from build123d import *

# Parameters (mm, degrees)
SKETCH1_W           = 95.25
SKETCH1_H           = 247.65
BOSS_EXTRUDE1_DEPTH = 6.35
SKETCH2_R           = 38.1
CUT_EXTRUDE1_DEPTH  = 7.35
SKETCH3_W           = 6.35
SKETCH3_H           = 12.7
CUT_EXTRUDE2_DEPTH  = 7.35
LPATTERN1_COUNT     = 6
LPATTERN1_PITCH     = 25.4
SKETCH4_W           = 12.7
SKETCH4_H           = 6.35
CUT_EXTRUDE3_DEPTH  = 7.35
SKETCH5_W           = 12.7
SKETCH5_H           = 6.35
CUT_EXTRUDE4_DEPTH  = 7.35
SKETCH8_W           = 12.7
SKETCH8_H           = 6.881389346
CUT_EXTRUDE5_DEPTH  = 7.35
SKETCH9_R           = 1.75
CUT_EXTRUDE6_DEPTH  = 7.35
CIRPATTERN1_COUNT   = 4
FILLET1_R           = 12.7
SKETCH10_R          = 1.75
CUT_EXTRUDE7_DEPTH  = 7.35
CIRPATTERN2_COUNT   = 4


with BuildPart() as part:
    # Sketch1 → Boss-Extrude1 (new body)
    with BuildSketch(Plane(origin=(0, 0, 0), x_dir=(1, 0, 0), z_dir=(0, 1, 0))):
        with Locations((47.625, 123.825)):
            Rectangle(SKETCH1_W, SKETCH1_H)
    extrude(amount=BOSS_EXTRUDE1_DEPTH)

    # Sketch2 → Cut-Extrude1 (cut, through all)
    with BuildSketch(Plane(origin=(0, 6.35, 0), x_dir=(1, 0, 0), z_dir=(0, 1, 0))):
        with Locations((47.625, 200.025)):
            Circle(SKETCH2_R)
        with Locations((47.625, 47.625)):
            Circle(SKETCH2_R)
    extrude(amount=-CUT_EXTRUDE1_DEPTH, mode=Mode.SUBTRACT)

    # Sketch3 → Cut-Extrude2 (cut, through all)
    with BuildSketch(Plane(origin=(0, 6.35, 0), x_dir=(1, 0, 0), z_dir=(0, 1, 0))):
        with Locations((3.175, 6.35)):
            Rectangle(SKETCH3_W, SKETCH3_H)
        with Locations((92.075, 6.35)):
            Rectangle(SKETCH3_W, SKETCH3_H)
    cut_extrude2 = extrude(amount=-CUT_EXTRUDE2_DEPTH, mode=Mode.SUBTRACT)

    # LPattern1: Cut-Extrude2 ×6
    with Locations(*[(0, 0, -i * LPATTERN1_PITCH) for i in range(1, LPATTERN1_COUNT)]):
        add(cut_extrude2, mode=Mode.SUBTRACT)

    # Sketch4 → Cut-Extrude3 (cut, through all)
    with BuildSketch(Plane(origin=(0, 6.35, 0), x_dir=(1, 0, 0), z_dir=(0, 1, 0))):
        with Locations((47.625, 3.175)):
            Rectangle(SKETCH4_W, SKETCH4_H)
        with Locations((22.225, 3.175)):
            Rectangle(SKETCH4_W, SKETCH4_H)
        with Locations((73.025, 3.175)):
            Rectangle(SKETCH4_W, SKETCH4_H)
    extrude(amount=-CUT_EXTRUDE3_DEPTH, mode=Mode.SUBTRACT)

    # Sketch5 → Cut-Extrude4 (cut, through all)
    with BuildSketch(Plane(origin=(0, 6.35, 0), x_dir=(1, 0, 0), z_dir=(0, 1, 0))):
        with Locations((22.225, 92.075)):
            Rectangle(SKETCH5_W, SKETCH5_H)
        with Locations((47.625, 92.075)):
            Rectangle(SKETCH5_W, SKETCH5_H)
        with Locations((73.025, 92.075)):
            Rectangle(SKETCH5_W, SKETCH5_H)
    extrude(amount=-CUT_EXTRUDE4_DEPTH, mode=Mode.SUBTRACT)

    # Sketch8 → Cut-Extrude5 (cut, through all)
    with BuildSketch(Plane(origin=(0, 6.35, 0), x_dir=(1, 0, 0), z_dir=(0, 1, 0))):
        with Locations((22.225, 116.170967205)):
            Rectangle(SKETCH8_W, SKETCH8_H)
        with Locations((47.625, 116.170967205)):
            Rectangle(SKETCH8_W, SKETCH8_H)
        with Locations((73.025, 116.170967205)):
            Rectangle(SKETCH8_W, SKETCH8_H)
    extrude(amount=-CUT_EXTRUDE5_DEPTH, mode=Mode.SUBTRACT)

    # Sketch9 → Cut-Extrude6 (cut, through all)
    with BuildSketch(Plane(origin=(0, 6.35, 0), x_dir=(1, 0, 0), z_dir=(0, 1, 0))):
        with Locations((12.7, 82.55)):
            Circle(SKETCH9_R)
    cut_extrude6 = extrude(amount=-CUT_EXTRUDE6_DEPTH, mode=Mode.SUBTRACT)

    # CirPattern1: Cut-Extrude6 ×4 about axis
    cirpattern1_axis = Axis((47.625, 0, -47.625), (0, 1, 0))
    for i in range(1, CIRPATTERN1_COUNT):
        add(cut_extrude6.rotate(cirpattern1_axis, i * 360 / CIRPATTERN1_COUNT), mode=Mode.SUBTRACT)

    # Fillet1
    fillet1_edges = [part.edges().sort_by_distance(p)[0] for p in [
        (0, 3.175, -247.65),
        (95.25, 3.175, -247.65),
    ]]
    fillet(fillet1_edges, radius=FILLET1_R)

    # Sketch10 → Cut-Extrude7 (cut, through all)
    with BuildSketch(Plane(origin=(0, 6.35, 0), x_dir=(1, 0, 0), z_dir=(0, 1, 0))):
        with Locations((12.7, 234.95)):
            Circle(SKETCH10_R)
    cut_extrude7 = extrude(amount=-CUT_EXTRUDE7_DEPTH, mode=Mode.SUBTRACT)

    # CirPattern2: Cut-Extrude7 ×4 about axis
    cirpattern2_axis = Axis((47.625, 0, -200.025), (0, 1, 0))
    for i in range(1, CIRPATTERN2_COUNT):
        add(cut_extrude7.rotate(cirpattern2_axis, i * 360 / CIRPATTERN2_COUNT), mode=Mode.SUBTRACT)


solid = part.part
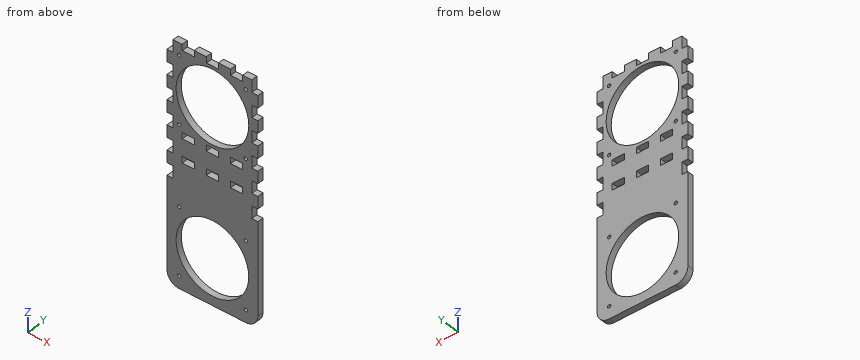
Source: CAD feature listing. Evaluate the final solid. Frame: model axes, mm. Round coordinates to 2 decimals unless told otherwise and drop trailing zeros. Order: outer loops, then holes, each group sorted by start corner. A loop starts at its lowest first (then second) coordinate and runs counter-clockwise, first axis right, second up. Notation, with made-up numbers: (8, -6.5) - (32, -6.5) arc R36 ccw to (32, 32.5) - close; hole circle Ø10 at (71, 45). An arc over 180 degrees is marked (long way). Use a Markdown table: item, result. Add a question column.
1. First-contact query: pin 1 (1.9 mm diameter, centred on x = 3, y = 2.5, fed in from +Z); pin 2 (3 mm diameter, centred on y = 3.5, z = -81, fed in from +X). Flat tips, straight axial feed; report the tip coordinate or a pass-through.
2. Section query C-C (z = -31). Return the cut outline in (x, y).
3. Section query A-A (x = 34.5). Return the cut outline in (y, z).
4. Section query B-B (z = -206.5). Return the cut outline in (x, y), then the cut area to 3 significant figures.
5. Section query D-D (y = 2.5). Give the number of separate pieces and of enclosed holes in the cut face, then the cut area to 3 significant figures.
6. Line query: probe 1 along X at (y, z) = (2.25, -113) (3 decimals); probe 2 along Z at (x, y) = (32.5, 5); probe 3 along X at (y, z) = (3.25, -165.1). Output: solid intervals per line, ascending.
Derived:
| question | item | result |
|---|---|---|
| 1 | pin 1 | z = -12.7 |
| 1 | pin 2 | x = 88.9 |
| 2 | outline | (6.35, 0) - (13.34, 0) - (13.34, 6.35) - (6.35, 6.35) - close; (81.91, 0) - (88.9, 0) - (88.9, 6.35) - (81.91, 6.35) - close |
| 3 | outline | (0, -247.65) - (6.35, -247.65) - (6.35, -235.79) - (0, -235.79) - close; (0, -164.26) - (6.35, -164.26) - (6.35, -83.39) - (0, -83.39) - close; (0, -11.86) - (6.35, -11.86) - (6.35, 0) - (0, 0) - close |
| 4 | outline | (0, 0) - (10.08, 0) - (10.08, 6.35) - (0, 6.35) - close; (85.17, 0) - (95.25, 0) - (95.25, 6.35) - (85.17, 6.35) - close |
| 4 | area | 128 mm2 |
| 5 | separate pieces | 1 |
| 5 | enclosed holes | 16 |
| 5 | area | 12,600 mm2 |
| 6 | probe 1 | 6.35 to 15.875, 28.575 to 41.275, 53.975 to 66.675, 79.375 to 88.9 |
| 6 | probe 2 | -247.65 to -234.99, -165.06 to -82.59, -12.66 to 0 |
| 6 | probe 3 | 0 to 10.95, 14.45 to 32.4, 62.85 to 80.8, 84.3 to 95.25 |
